Design review of the part built by this model. Coordinates are the model's own, in mm. A direction names the side the tool comes from. Round coordinates to 2 decimals unless told otherwise and drop trailing zeros. Loops run counter-clockwise (first coordinate to the right, second up) from the corner with the lowest first, then second, coordinate; pieces in that order, holes last. Notation, with made-up numbers: (56, 17.5) -> (97, 17.5) arc R27 cw to (97, 53.5) -> close; hole circle Ø4 at (-33, 30.5). An arc over 180 degrees is marked (long way). Use a Markdown table: item, result. Add a question column.
from build123d import *

# Parameters (mm, degrees)
F0_R     = 13.156852
F1_DEPTH = 247.65
F2_W     = 26.60638
F2_H     = 36.989354
F3_DEPTH = 65.532
F4_R     = 12.7
F5_R     = 12.7
F6_W     = 214.072559
F6_H     = 7.634542
F7_DEPTH = 11.43
F8_W     = 215.813644
F8_H     = 7.254239
F9_DEPTH = 8.89


with BuildPart() as f1:
    # F0 (on Front) → F1 (new body)
    with BuildSketch(Plane.XZ):
        Circle(F0_R)
    extrude(amount=F1_DEPTH)

    # F2 (on Top) → F3 (join)
    with BuildSketch(Plane.XY):
        with Locations((-0.648935, -126.607973)):
            Rectangle(F2_W, F2_H)
    extrude(amount=F3_DEPTH)

    # F4
    f4_edges = [f1.edges().sort_by_distance(p)[0] for p in [
        (-13.156852, -247.65, 0),
    ]]
    fillet(f4_edges, radius=F4_R)

    # F5
    f5_edges = [f1.edges().sort_by_distance(p)[0] for p in [
        (-13.156852, 0, 0),
    ]]
    fillet(f5_edges, radius=F5_R)

    # F6 (on Right) → F7 (join)
    with BuildSketch(Plane.YZ):
        with Locations((-123.286945, 0)):
            Rectangle(F6_W, F6_H)
    extrude(amount=-F7_DEPTH)

    # F8 (on Right) → F9 (join)
    with BuildSketch(Plane.YZ):
        with Locations((-124.603193, -0.566737)):
            Rectangle(F8_W, F8_H)
    extrude(amount=F9_DEPTH)


solid = f1.part
1. To check wall thickness, follow probe 1 along Y at (x, z) = (0, 17.5); probe 2 along Z at (x, y) = (0.75, -163.5); probe 3 along Z at (x, y) = (-7.25, -54). State the ranges of each line that lie inside material, in increasing order. Write a range as from..to.
2. Consider section A-A on z = 34. State the section outline as (x, y) points.
3. Insertion check: P1, Ø1, axis at x = -1, y = -66.5, coming from the +Z side; P2, Ø4, axis at y = -219.5, z = 2.5, coming from the -X side; P3, Ø8, axis at x = -9.5, z = 3, coming from the -Y side. Each pin has a flat end and moves straight along its axis. Give the tip position at first contact, or say it passes through.
4. For faces 1 (the face through (6.071, -122.269, -11.672)), 2 (the face through (-13.952, -127, 32)), 3 (the face through (12.654, -127, 34)), list the 3-axis set-ups (+Z, -Z, +X, -X, +Y, -Y) from which the entire face can be reached by the end or side of a thin tool; tool diameter is ignored.
5. Consider section B-B on y = -52. State the section outline as (x, z) points.
Verdict:
| question | item | result |
|---|---|---|
| 1 | probe 1 | y = -145.1..-108.11 |
| 1 | probe 2 | z = -13.14..13.14 |
| 1 | probe 3 | z = -10.98..10.98 |
| 2 | outline | (-13.95, -145.1) -> (12.65, -145.1) -> (12.65, -108.11) -> (-13.95, -108.11) -> close |
| 3 | P1 | stops at z = 13.15 |
| 3 | P2 | stops at x = -13.15 |
| 3 | P3 | stops at y = -246.39 |
| 4 | face 1 | none |
| 4 | face 2 | +Z, -Z, -X, +Y, -Y |
| 4 | face 3 | +Z, +X, +Y, -Y |
| 5 | outline | circle Ø26.31 at (0, 0) |
